Geometry: final body of the model. Coordinates: model frame, mm. A direction names the side the tool comes from. Coordinates: 2 decimals unless noted, no trailing zeros. Write each loop counter-clockwise with the first axis right and the second up, starting at its lowest first coordinate (ties: lowest second). Pieces come first, ordered by that corner, then holes. Notation, with made-up numbers: M -19.75,36.25 L 25.25,36.25 A16 cw 25.25,56.25 Z; hole C 57.25,70 d8. An arc over 180 degrees is marked long. Write item = value, one per line. Start each with the question number.
Item 1: Reachability of faces 5 (the flat face through (25, -13, -2)), 6 (the flat face through (21, -5, -3)), 7 (the flat face through (25, 2.5, -2)) from +Z, -Z, +X, -X, +Y, -Y: full face, straight path, thin tool, end or side. Return the list, or none.
Item 2: Pull-direction query (Y, two-part tool) for faces 1 (the cylindrical face through (14.36, -16.55, 0.74)), 2 (the cylindrical face through (20.85, -17.13, 0.74)), 3 (the flat face through (16, -12, 1.5)), 4 (the cylindrical face through (25.4, -9.7, -2.4)); classes: +Y half, -Y half, draft (parallel to the pull), parting line (faces both ways), or undercut.
Item 3: Section B-B on z = -1.75. Output: boundary loops of the cut face in (x, y).
Item 4: Section C-C on y = -15.5. Output: boundary loops of the cut face in (x, z), plus the area to 3 significant figures.
Item 5: Section A-A on x = 24.5. Output: boundary loops of the cut face in (y, z), plus the area to 3 significant figures.
Item 6: First-contact query: pin 1 Ø4 at (x, z) = (24.5, -2) entering from -Y; pin 2 Ø3 at (x, y) = (11.5, -11.5) entering from -Z; pin 3 Ø3 at (x, z) = (4.5, 0.5) entering from +Y; pin 4 Ø2 at (x, y) = (24.5, -10) entering from -Z. Flat tips, straight axial feed; report the tip coordinate or a pass-through.
Item 7: Ray query, L1, parallel to Y at x = 24.5, z = -2; L2, parallel to Y at x = 28, z = 0.5; L3, parallel to Z at x = 18, y = -16. Return the intervals inside material, ascending. Write a range as [from, to].
Item 8: Section D-D on x = 15.5. Output: boundary loops of the cut face in (y, z), plus the area to 3 significant figures.
Autodesk Inventor part; units mm, degrees
ref_plane "YZ Plane" through (0, 0, 0) normal (1, 0, 0) x (0, 1, 0)
ref_plane "XZ Plane" through (0, 0, 0) normal (0, 1, 0) x (-1, 0, 0)
ref_plane "XY Plane" through (0, 0, 0) normal (0, 0, 1) x (1, 0, 0)
sketch "Sketch1" plane through (0, 0, 0) normal (0, 0, 1) x (1, 0, 0)
  line L0 (20.0607, 17.4322) -> (17.4322, 20.0607)
  arc A0 (17.4322, 20.0607) -> (16.3716, 20.5) centre (16.3716, 19) ccw
  line L1 (16.3716, 20.5) -> (-16.3716, 20.5)
  arc A1 (-16.3716, 20.5) -> (-17.4322, 20.0607) centre (-16.3716, 19) ccw
  line L2 (-17.4322, 20.0607) -> (-20.0607, 17.4322)
  arc A2 (-20.0607, 17.4322) -> (-20.5, 16.3716) centre (-19, 16.3716) ccw
  line L3 (-20.5, 16.3716) -> (-20.5, -16.3716)
  arc A3 (-20.5, -16.3716) -> (-20.0607, -17.4322) centre (-19, -16.3716) ccw
  line L4 (-20.0607, -17.4322) -> (-17.4322, -20.0607)
  arc A4 (-17.4322, -20.0607) -> (-16.3716, -20.5) centre (-16.3716, -19) ccw
  line L5 (-16.3716, -20.5) -> (16.3716, -20.5)
  arc A5 (16.3716, -20.5) -> (17.4322, -20.0607) centre (16.3716, -19) ccw
  line L6 (17.4322, -20.0607) -> (20.0607, -17.4322)
  arc A6 (20.0607, -17.4322) -> (20.5, -16.3716) centre (19, -16.3716) ccw
  line L7 (20.5, -16.3716) -> (20.5, 16.3716)
  arc A7 (20.5, 16.3716) -> (20.0607, 17.4322) centre (19, 16.3716) ccw
  circle A8 centre (0, 0) radius 16.5
  circle A9 centre (15.5, 15.5) radius 1.55
  circle A10 centre (15.5, -15.5) radius 1.55
  circle A11 centre (-15.5, -15.5) radius 1.55
  circle A12 centre (-15.5, 15.5) radius 1.55
  line L8 (0, -13) -> (0, -16)
  line L9 (0, -13) -> (-1.914, -11.086)
  arc A13 (-11.25, 0) -> (-1.914, -11.086) centre (0, 0) ccw
  line L10 (-11.25, 0) -> (-11.25, -10.75)
  line L11 (-11.25, -10.75) -> (-21, -10.75)
  line L12 (-21, -10.75) -> (-21, -21)
  line L13 (-21, -21) -> (-5, -21)
  line L14 (-5, -21) -> (0, -16)
  circle A14 centre (-15.5, -15.5) radius 2.8
  line L15 (20.5, -5.5) -> (15.5563, -5.5)
  line L16 (21, 16.3716) -> (21, -16.3716)
  line L17 (21, -16.3716) -> (20.5, -16.3716)
  arc A15 (20.4142, -17.7858) -> (21, -16.3716) centre (19, -16.3716) ccw
  line L18 (20.4142, -17.7858) -> (17.7858, -20.4142)
  arc A16 (16.3716, -21) -> (17.7858, -20.4142) centre (16.3716, -19) ccw
  line L19 (16.3716, -21) -> (-16.3716, -21)
  line L20 (20.5, -5.5) -> (21, -5.5)
  point P0 (0, 0)
  point P1 (-0.4926, -16.4926)
  point P2 (-4.5, -20.5)
extrude "Extrusion1" add sketch "Sketch1" along normal blind 1.5 contours L20 L16 L17 L7 | L7 A6 L6 A5 L5 L14 A8 L15 | L17 A15 L18 A16 L19 L14 L5 A5 L6 A6
sketch "Sketch2" plane through (0, 0, 1.5) normal (0, 0, 1) x (1, 0, 0)
  circle A0 centre (24.5, -10) radius 0.95
  circle A1 centre (24.5, -0.5) radius 0.95
  line L0 (30, 2.5) -> (21, 2.5)
  line L1 (21, 2.5) -> (21, -13)
  line L2 (21, -13) -> (30, -13)
  line L3 (30, -13) -> (30, 2.5)
  point P0 (0, 0)
  point P1 (21, -5.5)
  dimension "d4" = 24.5
  dimension "d5" = 24.5
  dimension "d6" = 9.5
  dimension "d7" = 1.9
  dimension "d8" = 1.9
  dimension "d9" = 10
  dimension "d10" = 3
  dimension "d11" = 9
  dimension "d12" = 3
extrude "Extrusion2" add sketch "Sketch2" against normal blind 8
sketch "Sketch3" plane through (0, 0, 1.5) normal (0, 0, 1) x (1, 0, 0)
  arc A0 (-0.4926, -16.4926) -> (15.5563, -5.5) centre (0, 0) ccw
  circle A1 centre (24.5, -0.5) radius 0.95
  circle A2 centre (24.5, -10) radius 0.95
  line L0 (-0.4926, -16.4926) -> (-5, -21)
  line L1 (-5, -21) -> (16.3716, -21)
  arc A3 (16.3716, -21) -> (17.7858, -20.4142) centre (16.3716, -19) ccw
  line L2 (17.7858, -20.4142) -> (20.4142, -17.7858)
  arc A4 (20.4142, -17.7858) -> (21, -16.3716) centre (19, -16.3716) ccw
  line L3 (21, 2.5) -> (21, -5.5)
  line L4 (21, -13) -> (30, -13)
  line L5 (30, -13) -> (30, 2.5)
  line L6 (30, 2.5) -> (21, 2.5)
  line L7 (21, -5.5) -> (15.5563, -5.5)
  arc A5 (-0.4926, -16.4926) -> (15.5563, -5.5) centre (0, 0) ccw
  circle A6 centre (15.5, -15.5) radius 1.55
  circle A7 centre (0, 0) radius 16.5
  line L8 (21, 2.5) -> (16.3095, 2.5)
  line L9 (21, -13) -> (30, -13)
  line L10 (22.3286, -13) -> (17.1369, -20.8478)
  arc A8 (16.3716, -21) -> (17.7858, -20.4142) centre (16.3716, -19) ccw
  line L11 (21, -16.3716) -> (21, -13)
  point P0 (0, 0)
  point P1 (21, -17)
  point P2 (15.5563, -5.5)
  point P3 (17.2535, -20.795)
  point P4 (17.9687, -20.2313)
extrude "Extrusion3" add sketch "Sketch3" against normal blind 1.5 contours A7 L8 L3 L7
properties part number "Y-LIMIT SWITCH PLATE"
Responses:
q1.face_5 = +Z, -Z, +X, -Y
q1.face_6 = -Z, -X, +Y, -Y
q1.face_7 = +Z, -Z, +X, -X, +Y
q2.face_1 = undercut
q2.face_2 = -Y half
q2.face_3 = draft
q2.face_4 = undercut
q3.outline = M 21,-13 L 30,-13 L 30,2.5 L 21,2.5 Z; hole C 24.5,-10 d1.9; hole C 24.5,-0.5 d1.9
q4.outline = M 5.66,0 L 13.95,0 L 13.95,1.5 L 5.66,1.5 Z; M 17.05,0 L 21,0 L 21,1.5 L 17.05,1.5 Z
q4.area = 18.4 mm²
q5.outline = M -13,-6.5 L -10.95,-6.5 L -10.95,1.5 L -13,1.5 Z; M -9.05,-6.5 L -1.45,-6.5 L -1.45,1.5 L -9.05,1.5 Z; M 0.45,-6.5 L 2.5,-6.5 L 2.5,1.5 L 0.45,1.5 Z
q5.area = 93.6 mm²
q6.pin_1 = -13
q6.pin_2 = 0
q6.pin_3 = -15.37
q6.pin_4 = -6.5
q7.L1 = [-13, -10.95], [-9.05, -1.45], [0.45, 2.5]
q7.L2 = [-13, 2.5]
q7.L3 = [0, 1.5]
q8.outline = M -21,0 L -17.05,0 L -17.05,1.5 L -21,1.5 Z; M -13.95,0 L -5.66,0 L -5.66,1.5 L -13.95,1.5 Z
q8.area = 18.4 mm²
